Part model, mm, in its own coordinate system. Round coordinates to 2 decimals unless told otherwise and drop trailing zeros. Order: outer loops, then holes, each group sorted by start corner. A loop starts at its lowest first (then second) coordinate and runs counter-clockwise, first axis right, second up. Notation, with made-up numbers: (47.5, 39) -> (105.5, 39) arc R17 ccw to (105.5, 70) -> close; hole circle Ø4 at (24.5, 74). An arc over 180 degrees is marked (long way). Return JSON: item names as keys, results as strings. Group by question number.
from build123d import *

# Parameters (mm, degrees)
ESQUISSE1_W             = 20
ESQUISSE1_H             = 40
ESQUISSE1_R             = 3.974062066
BOSS_EXTRU_1_DEPTH      = 10
ESQUISSE2_R             = 1.4
ENL_V_MAT_EXTRU_1_DEPTH = 28


with BuildPart() as part:
    # Esquisse1 → Boss.-Extru.1 (new body)
    with BuildSketch(Plane.XY):
        Rectangle(ESQUISSE1_W, ESQUISSE1_H)
        with Locations((0, 12)):
            Circle(ESQUISSE1_R, mode=Mode.SUBTRACT)
        with Locations((0, -12)):
            Circle(ESQUISSE1_R, mode=Mode.SUBTRACT)
    extrude(amount=BOSS_EXTRU_1_DEPTH)

    # Esquisse2 → Enlèv. mat.-Extru.1 (cut)
    with BuildSketch(Plane.ZY.offset(10)):
        with Locations((5, 12)):
            Circle(ESQUISSE2_R)
        with Locations((5, -12)):
            Circle(ESQUISSE2_R)
    extrude(amount=-ENL_V_MAT_EXTRU_1_DEPTH, mode=Mode.SUBTRACT)


solid = part.part
(1) Mould opens along Z. For faces 1 (the cylindrical face through (6.82, -10.82, 5.75)), 2 (the flat face through (10, 0, 5)), 3 (the flat face through (0, 0, 0)) say: pulls with the +Z half, pulls with the -Z half, needs draft (parallel to the pull), parting line crosses it, or undercut.
(2) Pin check, flat tips, straight feed: P1, Ø4.5, axis at y = -12, z = 5, coming from the +X side; P2, Ø2, axis at x = 1, y = -10.5, coming from the +Z side. Stop position of each tip, or through.
(3) Saw through at C-C, the plane y = -12. List the corners of the cut face in (x, z).
(4) Saw through at D-D, the plane x = 8.5. List the corners of the cut face in (y, z), and give its area (3 significant figures).
(5) Probe L1, parallel to Y at x = 8.5, z = 5; L2, parallel to Y at x = 0, z = 6; L3, parallel to X at y = -12, z = 8.25. List the from-to ranges inside material, lowest first. Write a range as [from, to].
(6) Saw through at A-A, the plane x = 0. List the corners of the cut face in (y, z).
(7) Saw through at B-B, the plane z = 5. List the corners of the cut face in (x, y).
Results are:
{
 "1": {"face 1": "undercut", "face 2": "needs draft", "face 3": "pulls with the -Z half"},
 "2": {"P1": "stops at x = 10", "P2": "passes through"},
 "3": {"outline": "(-10, 0) -> (-3.97, 0) -> (-3.97, 3.6) -> (-10, 3.6) -> close; (-10, 6.4) -> (-3.97, 6.4) -> (-3.97, 10) -> (-10, 10) -> close; (3.97, 0) -> (10, 0) -> (10, 3.6) -> (3.97, 3.6) -> close; (3.97, 6.4) -> (10, 6.4) -> (10, 10) -> (3.97, 10) -> close"},
 "4": {"outline": "(-20, 0) -> (20, 0) -> (20, 10) -> (-20, 10) -> close; hole circle Ø2.8 at (-12, 5); hole circle Ø2.8 at (12, 5)", "area": "388 mm^2"},
 "5": {"L1": "y = [-20, -13.4], [-10.6, 10.6], [13.4, 20]", "L2": "y = [-20, -15.97], [-8.03, 8.03], [15.97, 20]", "L3": "x = [-10, -3.97], [3.97, 10]"},
 "6": {"outline": "(-20, 0) -> (-15.97, 0) -> (-15.97, 10) -> (-20, 10) -> close; (-8.03, 0) -> (8.03, 0) -> (8.03, 10) -> (-8.03, 10) -> close; (15.97, 0) -> (20, 0) -> (20, 10) -> (15.97, 10) -> close"},
 "7": {"outline": "(-10, -20) -> (10, -20) -> (10, -13.4) -> (3.72, -13.4) arc R3.97 cw to (-3.72, -13.4) -> (-10, -13.4) -> close; (-10, -10.6) -> (-3.72, -10.6) arc R3.97 cw to (3.72, -10.6) -> (10, -10.6) -> (10, 10.6) -> (3.72, 10.6) arc R3.97 cw to (-3.72, 10.6) -> (-10, 10.6) -> close; (-10, 13.4) -> (-3.72, 13.4) arc R3.97 cw to (3.72, 13.4) -> (10, 13.4) -> (10, 20) -> (-10, 20) -> close"}
}
